```python
from build123d import *

# Parameters (mm, degrees)
SKETCH1_W           = 80
SKETCH1_H           = 50
BOSS_EXTRUDE1_DEPTH = 10
SKETCH2_W           = 10
SKETCH2_H           = 10
BOSS_EXTRUDE2_DEPTH = 10
SKETCH3_W           = 10
SKETCH3_H           = 10
CUT_EXTRUDE1_DEPTH  = 5
SKETCH4_R           = 3
CUT_EXTRUDE2_DEPTH  = 5
SKETCH5_W           = 10
SKETCH5_H           = 10
BOSS_EXTRUDE3_DEPTH = 10
SKETCH6_W           = 10
SKETCH6_H           = 10
CUT_EXTRUDE3_DEPTH  = 5
SKETCH7_R           = 3
CUT_EXTRUDE4_DEPTH  = 5
SKETCH10_W          = 10
SKETCH10_H          = 50
BOSS_EXTRUDE4_DEPTH = 70
SKETCH11_W          = 50
SKETCH11_H          = 51
CUT_EXTRUDE5_DEPTH  = 5
SKETCH12_R          = 1.5
CUT_EXTRUDE7_DEPTH  = 10


with BuildPart() as part:
    # Sketch1 → Boss-Extrude1 (new body)
    with BuildSketch(Plane(origin=(0, 0, 0), x_dir=(1, 0, 0), z_dir=(0, 1, 0))):
        with Locations((13.76, -10.152)):
            Rectangle(SKETCH1_W, SKETCH1_H)
    extrude(amount=BOSS_EXTRUDE1_DEPTH)

    # Sketch2 → Boss-Extrude2 (add)
    with BuildSketch(Plane.XY.offset(35.152)):
        with Locations((-21.24, 5)):
            Rectangle(SKETCH2_W, SKETCH2_H)
    extrude(amount=BOSS_EXTRUDE2_DEPTH)

    # Sketch3 → Cut-Extrude1 (cut)
    with BuildSketch(Plane(origin=(0, 10, 0), x_dir=(1, 0, 0), z_dir=(0, 1, 0))):
        with Locations((-21.24, -40.152)):
            Rectangle(SKETCH3_W, SKETCH3_H)
    extrude(amount=-CUT_EXTRUDE1_DEPTH, mode=Mode.SUBTRACT)

    # Sketch4 → Cut-Extrude2 (cut)
    with BuildSketch(Plane(origin=(0, 5, 0), x_dir=(1, 0, 0), z_dir=(0, 1, 0))):
        with Locations((-21.24, -40.152)):
            Circle(SKETCH4_R)
    extrude(amount=-CUT_EXTRUDE2_DEPTH, mode=Mode.SUBTRACT)

    # Sketch5 → Boss-Extrude3 (add)
    with BuildSketch(Plane(origin=(0, 0, -14.848), x_dir=(-1, 0, 0), z_dir=(0, 0, -1))):
        with Locations((21.24, 5)):
            Rectangle(SKETCH5_W, SKETCH5_H)
    extrude(amount=BOSS_EXTRUDE3_DEPTH)

    # Sketch6 → Cut-Extrude3 (cut)
    with BuildSketch(Plane(origin=(0, 10, 0), x_dir=(1, 0, 0), z_dir=(0, 1, 0))):
        with Locations((-21.24, 19.848)):
            Rectangle(SKETCH6_W, SKETCH6_H)
    extrude(amount=-CUT_EXTRUDE3_DEPTH, mode=Mode.SUBTRACT)

    # Sketch7 → Cut-Extrude4 (cut)
    with BuildSketch(Plane(origin=(0, 5, 0), x_dir=(1, 0, 0), z_dir=(0, 1, 0))):
        with Locations((-21.24, 19.848)):
            Circle(SKETCH7_R)
    extrude(amount=-CUT_EXTRUDE4_DEPTH, mode=Mode.SUBTRACT)

    # Sketch10 → Boss-Extrude4 (add)
    with BuildSketch(Plane(origin=(0, 10, 0), x_dir=(1, 0, 0), z_dir=(0, 1, 0))):
        with Locations((48.76, -10.152)):
            Rectangle(SKETCH10_W, SKETCH10_H)
    extrude(amount=BOSS_EXTRUDE4_DEPTH)

    # Sketch11 → Cut-Extrude5 (cut)
    with BuildSketch(Plane(origin=(53.76, 0, 0), x_dir=(0, 0, -1), z_dir=(1, 0, 0))):
        with Locations((-10.152, 54.5)):
            Rectangle(SKETCH11_W, SKETCH11_H)
    extrude(amount=-CUT_EXTRUDE5_DEPTH, mode=Mode.SUBTRACT)

    # Sketch12 → Cut-Extrude7 (cut)
    with BuildSketch(Plane(origin=(48.76, 0, 0), x_dir=(0, 0, -1), z_dir=(1, 0, 0))):
        with Locations((-10.152, 54.5)):
            Circle(SKETCH12_R)
    extrude(amount=-CUT_EXTRUDE7_DEPTH, mode=Mode.SUBTRACT)


solid = part.part
```
The listing builds one solid part. Answer for the finished solid, in the listing's coordinates (mm). A direction names the side the tool comes from. Coordinates: 2 decimals unless noted, no trailing zeros. Loops run counter-clockwise (first coordinate to the right, second up) from the corner with the lowest first, then second, coordinate; pieces in that order, holes last. Notation, with made-up numbers: (83.25, 45) -> (104.25, 45) arc R28 ccw to (104.25, 84) -> close; hole circle Ø7 at (-7.75, -29.75). An arc over 180 degrees is marked (long way). Use one line per item in the form item = value. Start each with the question number.
Item 1: The mould has two halves that part along Y. Classify faces 4 (the face through (46.3, 53.17, 9.46)), 5 (the face through (14, 0, 11)), 6 (the face through (9, 10, 11)), 7 (the face through (25, 7, -14.848)): released by +Y, released by -Y, zero draft, split by the parting line, or undercut.
Item 2: The part is cut by section A-A on x = -21.24. Determine the outline of the cut face in (y, z), then the cut area to 3 significant figures.
Item 3: The part is cut by section C-C on z = -9. Determine the outline of the cut face in (x, y), then the cut area to 4 significant figures.
Item 4: The part is cut by section D-D on x = 45.5. Determine the outline of the cut face in (y, z).
Item 5: Consider L1, parallel to Z at x = -21.24, y = 2.3; L2, parallel to Z at x = -21, y = 3; L3, parallel to X at y = 47.5, z = 20.5. Determine where each line is inside the solid, lowest interval first. Write a range as [from, to].
Item 6: Flat-ended cylindrical pins translate along their axes: pin 1 Ø1.5 at (y, z) = (1.5, -21.5) entering from +X; pin 2 Ø3 at (x, z) = (-23, -22) entering from +Y; pin 3 Ø3 at (y, z) = (49.5, 1) entering from +X; pin 4 Ø10 at (x, z) = (26, 31.5) entering from -Y. Find the tip coordinate at first contact, or state that the pin passes through.
Item 7: The part is cut by section B-B on y = 54.5. Determine the outline of the cut face in (x, z), then the cut area to 3 significant figures.
Item 8: A tool of negligible diameter and unlimited length cuts with its end or side. For faces 1 (the face through (-16.24, 2, 40)), 2 (the face through (-24, 5, -22)), 3 (the face through (48.76, 55, 16)), from which of +Z, -Z, +X, -X, +Y, -Y can it reach the whole face along a straight path? Write none if from no direction.
Answer key:
q1.face_4 = undercut
q1.face_5 = released by -Y
q1.face_6 = released by +Y
q1.face_7 = zero draft
q2.outline = (0, -24.85) -> (5, -24.85) -> (5, -22.85) -> (0, -22.85) -> close; (0, -16.85) -> (5, -16.85) -> (5, -14.85) -> (10, -14.85) -> (10, 35.15) -> (5, 35.15) -> (5, 37.15) -> (0, 37.15) -> close; (0, 43.15) -> (5, 43.15) -> (5, 45.15) -> (0, 45.15) -> close
q2.area = 540 mm2
q3.outline = (-26.24, 0) -> (53.76, 0) -> (53.76, 29) -> (48.76, 29) -> (48.76, 80) -> (43.76, 80) -> (43.76, 10) -> (-26.24, 10) -> close
q3.area = 1,245 mm2
q4.outline = (0, -14.85) -> (80, -14.85) -> (80, 35.15) -> (0, 35.15) -> close; hole circle Ø3 at (54.5, 10.15)
q5.L1 = [-24.85, -22.85], [-16.85, 37.15], [43.15, 45.15]
q5.L2 = [-24.85, -22.84], [-16.86, 37.16], [43.14, 45.15]
q5.L3 = [43.76, 48.76]
q6.pin_1 = -16.24
q6.pin_2 = 5
q6.pin_3 = 48.76
q6.pin_4 = 0
q7.outline = (43.76, -14.85) -> (48.76, -14.85) -> (48.76, 8.65) -> (43.76, 8.65) -> close; (43.76, 11.65) -> (48.76, 11.65) -> (48.76, 35.15) -> (43.76, 35.15) -> close
q7.area = 235 mm2
q8.face_1 = +Z, +X, +Y, -Y
q8.face_2 = -Z, +X, -X, +Y
q8.face_3 = +Z, -Z, +X, +Y
